The listing builds one solid part. Answer for the finished solid, in the listing's coordinates (mm). A direction names the side the tool comes from. Coordinates: 2 decimals unless noted, no trailing zeros. Write each loop counter-clockwise with the first axis right and the second up, starting at its lowest first coordinate (ties: lowest second). Pieces come first, ordered by that corner, then holes.
from build123d import *

# Parameters (mm, degrees)
SKETCH1_W           = 38.1
SKETCH1_H           = 381
BOSS_EXTRUDE2_DEPTH = 12.7
SKETCH3_R           = 3.175
CUT_EXTRUDE3_DEPTH  = 863.6
SKETCH4_R           = 3.175
CUT_EXTRUDE4_DEPTH  = 36
SKETCH2_R           = 3.175
CUT_EXTRUDE5_DEPTH  = 52.578
SKETCH5_R           = 3.175
CUT_EXTRUDE6_DEPTH  = 148.082


with BuildPart() as part:
    # Sketch1 → Boss-Extrude2 (new body)
    with BuildSketch(Plane.XY):
        Rectangle(SKETCH1_W, SKETCH1_H)
        with BuildLine():
            Line((19.05, 190.5), (120.463073453, 291.913073453))
            ThreePointArc((120.463073453, 291.913073453), (121.839580424, 298.833241309), (115.972945392, 302.753201513))
            Line((115.972945392, 302.753201513), (95.833457634, 302.753201513))
            ThreePointArc((95.833457634, 302.753201513), (93.403417839, 302.269836545), (91.343329574, 300.893329574))
            Line((91.343329574, 300.893329574), (-19.05, 190.5))
            Line((-19.05, 190.5), (19.05, 190.5))
        make_face()
    extrude(amount=BOSS_EXTRUDE2_DEPTH)

    # Sketch3 → Cut-Extrude3 (cut)
    with BuildSketch(Plane.XY.offset(12.7)):
        with Locations((95.396679576, 285.76176863)):
            Circle(SKETCH3_R)
    extrude(amount=-CUT_EXTRUDE3_DEPTH, mode=Mode.SUBTRACT)

    # Sketch4 → Cut-Extrude4 (cut)
    with BuildSketch(Plane.XY.offset(12.7)):
        Circle(SKETCH4_R)
    extrude(amount=-CUT_EXTRUDE4_DEPTH, mode=Mode.SUBTRACT)

    # Sketch2 → Cut-Extrude5 (cut)
    with BuildSketch(Plane.XY.offset(12.7)):
        with Locations((6.35, -177.8)):
            Circle(SKETCH2_R)
    extrude(amount=-CUT_EXTRUDE5_DEPTH, mode=Mode.SUBTRACT)

    # Sketch5 → Cut-Extrude6 (cut)
    with BuildSketch(Plane.XY.offset(12.7)):
        with Locations((0, 177.8)):
            Circle(SKETCH5_R)
    extrude(amount=-CUT_EXTRUDE6_DEPTH, mode=Mode.SUBTRACT)


solid = part.part
1. Find the intervals of material crossed by L1, parallel to X at y = 177.8, z = 5 (3 decimals); L2, parallel to Y at x = 0, z = 9.25 (3 decimals); L3, parallel to X at y = -177.8, z = 3 (3 decimals), in increasing order.
Results found:
L1: x = -19.05 to -3.175, 3.175 to 19.05
L2: y = -190.5 to -3.175, 3.175 to 174.625, 180.975 to 209.55
L3: x = -19.05 to 3.175, 9.525 to 19.05
2. Flat-ended cylindrical pins translate along their axes: P1, Ø6, axis at y = 45.5, z = 2, coming from the +X side; P2, Ø4, axis at x = 6.35, y = -177.8, coming from the +Z side; P3, Ø3, axis at x = 61, z = 7, coming from the +Y side; P4, Ø6, axis at x = 70, z = 9, coming from the +Y side. Find the tip coordinate at first contact, or state that the pin passes through.
Results found:
P1: stops at x = 19.05
P2: passes through
P3: stops at y = 272.05
P4: stops at y = 282.55
3. Section A-A on z = 10.25 is taken. Give the vertices of the cut face in (x, y) (3 decimals).
Results found:
outline: (-19.05, -190.5) - (19.05, -190.5) - (19.05, 190.5) - (120.463, 291.913) arc R6.35 ccw to (115.973, 302.753) - (95.833, 302.753) arc R6.35 ccw to (91.343, 300.893) - (-19.05, 190.5) - close; hole circle Ø6.35 at (0, 0); hole circle Ø6.35 at (0, 177.8); hole circle Ø6.35 at (6.35, -177.8); hole circle Ø6.35 at (95.397, 285.762)
4. A tool of negligible diameter and unlimited length cuts with its end or side. For faces 1 (the flat face through (19.05, -3, 6)), 2 (the flat face through (-19.05, -3, 6)), from which of +Z, -Z, +X, -X, +Y, -Y can it reach the whole face along a straight path? Write none if from no direction.
Results found:
face 1: +Z, -Z, +X, -Y
face 2: +Z, -Z, -X, +Y, -Y
5. Section B-B on y = 67 is taken. Give the vertices of the cut face in (x, z).
Results found:
outline: (-19.05, 0) - (19.05, 0) - (19.05, 12.7) - (-19.05, 12.7) - close
